from build123d import *

# Parameters (mm, degrees)
SKETCH1_W          = 25
SKETCH1_H          = 20
BASE_FLANGE1_DEPTH = 1
EDGE_FLANGE1_DEPTH = 20
EDGE_FLANGE2_DEPTH = 20
SKETCH15_W         = 50
SKETCH15_H         = 15
TAB1_DEPTH         = 1
SKETCH18_W         = 50
SKETCH18_H         = 15
TAB2_DEPTH         = 1


# Sheet-metal steps are written as plain solids
with BuildPart() as part:
    # Sketch1 → Base-Flange1 (new body)
    with BuildSketch(Plane(origin=(0, 0, 0), x_dir=(1, 0, 0), z_dir=(0, 1, 0))):
        Rectangle(SKETCH1_W, SKETCH1_H)
    extrude(amount=-BASE_FLANGE1_DEPTH)

    # Edge-Flange1 section (across the edge) → Edge-Flange1 (add)
    with BuildSketch(Plane(origin=(-14, 0, -10), x_dir=(1, 0, 0), z_dir=(0, 0, 1))):
        with BuildLine():
            Line((-1, 1.5), (-1, 20))
            Line((-1, 20), (0, 20))
            Line((0, 20), (0, 1.5))
            ThreePointArc((0, 1.5), (0.439339828, 0.439339828), (1.5, 0))
            Line((1.5, 0), (1.5, -1))
            ThreePointArc((1.5, -1), (-0.267766953, -0.267766953), (-1, 1.5))
        make_face()
    extrude(amount=EDGE_FLANGE1_DEPTH)

    # Edge-Flange2 section (across the edge) → Edge-Flange2 (add)
    with BuildSketch(Plane(origin=(14, 0, 10), x_dir=(-1, 0, 0), z_dir=(0, 0, -1))):
        with BuildLine():
            Line((-1, 1.5), (-1, 20))
            Line((-1, 20), (0, 20))
            Line((0, 20), (0, 1.5))
            ThreePointArc((0, 1.5), (0.439339828, 0.439339828), (1.5, 0))
            Line((1.5, 0), (1.5, -1))
            ThreePointArc((1.5, -1), (-0.267766953, -0.267766953), (-1, 1.5))
        make_face()
    extrude(amount=EDGE_FLANGE2_DEPTH)

    # Sketch15 → Tab1 (add)
    with BuildSketch(Plane(origin=(-14, 0, 0), x_dir=(0, 0, -1), z_dir=(1, 0, 0))):
        with Locations((-35, 12.5)):
            Rectangle(SKETCH15_W, SKETCH15_H)
    extrude(amount=-TAB1_DEPTH)

    # Sketch18 → Tab2 (add)
    with BuildSketch(Plane(origin=(15, 0, 0), x_dir=(0, 0, -1), z_dir=(1, 0, 0))):
        with Locations((-35, 12.5)):
            Rectangle(SKETCH18_W, SKETCH18_H)
    extrude(amount=-TAB2_DEPTH)


solid = part.part
Work out the finished part from the listing and answer in its coordinate system (mm). A direction names the side the tool comes from. Coordinates: 2 decimals unless noted, no trailing zeros. Write each loop counter-clockwise with the first axis right and the second up, starting at its lowest first coordinate (ties: lowest second). Pieces come first, ordered by that corner, then holes. Notation, with made-up numbers: M 78,-32.75 L 117,-32.75 A22 ccw 117,-18.75 Z; hole C -8.5,31 d4. An arc over 180 degrees is marked long. Write item = value, one per line.
1. The part is cut by section D-D (x = -4). Determine the outline of the cut face in (y, z).
Solution:
outline = M -1,-10 L 0,-10 L 0,10 L -1,10 Z
2. Determine the mould class of faces 4 (the face through (-15, 13, 25)), 5 (the face through (13.57, 0.45, 0.14)), 6 (the face through (0, -1, 0)), 7 (the face through (-13.57, 0.45, -0.14)) for opening direction X: released by +X, released by -X, zero draft, split by the parting line, or undercut.
Solution:
face_4 = released by -X
face_5 = undercut
face_6 = zero draft
face_7 = undercut
3. The part is cut by section A-A (y = 2.5). Determine the outline of the cut face in (x, z), then the cut area to 3 significant figures.
Solution:
outline = M -15,-10 L -14,-10 L -14,10 L -15,10 Z; M 14,-10 L 15,-10 L 15,10 L 14,10 Z
area = 40.0 mm2
4. The part is cut by section B-B (z = 29). Determine the outline of the cut face in (x, y).
Solution:
outline = M -15,5 L -14,5 L -14,20 L -15,20 Z; M 14,5 L 15,5 L 15,20 L 14,20 Z
5. For faces 1 (the face through (-0.1, -0.4, 10)), 2 (the face through (-14, 13, 25)), 3 (the face through (-14.248, -0.287, -0.14)), determine the directions among +Z, -Z, +X, -X, +Y, -Y from which every point of the face is accessible in a straight line to the end or side of a thin tool.
Solution:
face_1 = +Z, +X, -X, -Y
face_2 = +Z, -Z, +Y
face_3 = +Z, -Z, -X, -Y
6. Flat-ended cylindrical pins translate along their axes: pin 1 (4 mm diameter, centred on x = -2, z = 8.5, fed in from +Y); pin 2 (8 mm diameter, centred on x = -4, y = 5.5, fed in from +Z); pin 3 (0.5 mm diameter, centred on x = 14.5, z = 41, fed in from -Y); pin 4 (6.5 mm diameter, centred on x = 0, y = 1.5, fed in from +Z). Find the tip coordinate at first contact, or state that the pin passes through.
Solution:
pin_1 = 0
pin_2 = through
pin_3 = 5
pin_4 = 10
7. Straight lines are drawn through the part: line 1 (X direction, y = 16.25, z = 13.5); line 2 (Y direction, x = 6.25, z = 2). For each, find the intervals that lie inside material, in ascending order. Write a range as from..to.
Solution:
line_1 = -15..-14, 14..15
line_2 = -1..0
8. The part is cut by section C-C (z = -2.5). Determine the outline of the cut face in (x, y).
Solution:
outline = M -15,1.5 A2.5 ccw -12.5,-1 L 12.5,-1 A2.5 ccw 15,1.5 L 15,20 L 14,20 L 14,1.5 A1.5 cw 12.5,0 L -12.5,0 A1.5 cw -14,1.5 L -14,20 L -15,20 Z
